Model file for the job. Use its own axes, mm. A direction names the side the tool comes from. Round coordinates to 2 decimals unless told otherwise and drop trailing zeros. Loops run counter-clockwise (first coordinate to the right, second up) from the corner with the lowest first, then second, coordinate; pieces in that order, holes last. Notation, with made-up numbers: M 45.5,72.5 L 86.5,72.5 A18 cw 86.5,104.5 Z; hole C 15.25,51.5 d2. An arc over 180 degrees is marked long. Use a Markdown table: item, result. Add a question column.
Q1. Cut at C-C (z = -9.5). Give the cut face in (x, y), plus the area to 3 significant figures.
Q2. Cut at A-A (x = 12.5). Give the cut face in (y, z).
Q3. Pin check, flat tips, straight feed: pin 1 (5 mm diameter, centred on x = 0, z = 20.5, fed in from +Y); pin 2 (3 mm diameter, centred on x = 20.5, z = 0, fed in from -Y); pin 3 (1 mm diameter, centred on x = 16.5, y = 1.5, fed in from +Z); pin 4 (5 mm diameter, centred on x = 0, z = -9.5, fed in from -Y). Stop position of each tip, or through.
Q4. Probe line 1 (Z direction, x = 0, y = 1.4); line 2 (Z direction, x = 0, y = 1.6); line 3 (X direction, y = 1, z = -13). List the from-to ranges inside material, lowest first. Write a range as from..to.
Q5. Cut at D-D (z = 14). Give the cut face in (x, y).
Q6. Cut at B-B (y = 0.4). State how many separate pieces and enclosed holes the cut face has, plus the area to 3 significant figures.
Q7. Tool access for faces 1 (the face through (4, 2, 4)), 2 (the face through (-16, 1, -3)), 3 (the face through (-3, 1, 16)), 4 (the face through (22.6, 1.01, 2.14)), 5 (the face through (16, 1, -3)): list every direction of +Z, -Z, +X, -X, +Y, -Y with a clear straight run to the whole face (end or side of a thin tool).
Autodesk Inventor part; units mm, degrees
ref_plane "YZ Plane" through (0, 0, 0) normal (1, 0, 0) x (0, 1, 0)
ref_plane "XZ Plane" through (0, 0, 0) normal (0, 1, 0) x (-1, 0, 0)
ref_plane "XY Plane" through (0, 0, 0) normal (0, 0, 1) x (1, 0, 0)
sketch "Skizze1" plane through (0, 0, 0) normal (0, 1, 0) x (-1, 0, 0)
  line L0 (-23.5, -3) -> (23.5, -3)
  line L1 (23.5, -3) -> (23.5, 3)
  line L2 (23.5, 3) -> (-23.5, 3)
  line L3 (-23.5, 3) -> (-23.5, -3)
  line L4 (-23.5, -3) -> (23.5, 3) construction
  line L5 (23.5, -3) -> (-23.5, 3) construction
  line L6 (3, -23.5) -> (-3, -23.5)
  line L7 (-3, -23.5) -> (-3, 23.5)
  line L8 (-3, 23.5) -> (3, 23.5)
  line L9 (3, 23.5) -> (3, -23.5)
  line L10 (3, -23.5) -> (-3, 23.5) construction
  line L11 (-3, -23.5) -> (3, 23.5) construction
  point P0 (0, 0)
  dimension "d0" = 6
  dimension "d1" = 47
extrude "Extrusion1" add sketch "Skizze1" along normal blind 2
sketch "Skizze2" plane through (0, 0, 0) normal (0, -1, 0) x (1, 0, 0)
  circle A0 centre (0, 20.5) radius 1.6
  circle A1 centre (0, -20.5) radius 1.6
  circle A2 centre (20.5, 0) radius 1.6
  circle A3 centre (-20.5, 0) radius 1.6
  line L0 (0, 20.5) -> (0, -20.5) construction
  line L1 (3, -3) -> (3, -23.5) construction
  line L2 (20.5, 0) -> (-20.5, 0) construction
  circle A4 centre (0, 9.5) radius 1.6
  circle A5 centre (0, -9.5) radius 1.6
  circle A6 centre (12.5, 0) radius 1.6
  circle A7 centre (-12.5, 0) radius 1.6
  line L3 (0, 9.5) -> (0, -9.5) construction
  line L4 (12.5, 0) -> (-12.5, 0) construction
  point P0 (0, 0)
  point P1 (0, 0)
  dimension "d4" = 3.2
  dimension "d5" = 41
  dimension "d7" = 19
  dimension "d8" = 25
extrude "Extrusion2" cut sketch "Skizze2" against normal blind 2
fillet "Rundung1" radius 3 8 edges at (-3, 1, 23.5) (3, 1, 23.5) (23.5, 1, 3) (23.5, 1, -3) (3, 1, -23.5) (-3, 1, -23.5) (-23.5, 1, -3) (-23.5, 1, 3)
fillet "Rundung2" radius 8 4 edges at (3, 1, 3) (-3, 1, 3) (-3, 1, -3) (3, 1, -3)
sketch "Skizze3" plane through (0, 0, 0) normal (0, -1, 0) x (1, 0, 0)
  circle A0 centre (0, 0) radius 5
  dimension "d13" = 10
extrude "Extrusion3" cut sketch "Skizze3" against normal blind 2
chamfer "Fase1" distance 1 angle 45 8 edges at (-1.6, 0, 9.5) (-14.1, 0, 0) (10.9, 0, 0) (-1.6, 0, -9.5) (-1.6, 2, 20.5) (-22.1, 2, 0) (18.9, 2, 0) (-1.6, 2, -20.5)
equation "\"G_L\" = 0"
equation "\"G_H\" = 0"
equation "\"G_B\" = 0"
properties part number "Motorkreuz" material "GEDA Stahl"
Checked values:
| question | item | result |
|---|---|---|
| 1 | outline | M -3.14,0 L -2.6,0 L -1.6,1 L -1.6,2 L -3.14,2 Z; M 1.6,1 L 2.6,0 L 3.14,0 L 3.14,2 L 1.6,2 Z |
| 1 | area | 5.17 mm^2 |
| 2 | outline | M 0,-3 L 2,-3 L 2,-1.6 L 1,-1.6 L 0,-2.6 Z; M 0,2.6 L 1,1.6 L 2,1.6 L 2,3 L 0,3 Z |
| 3 | pin 1 | stops at y = 1.9 |
| 3 | pin 2 | passes through |
| 3 | pin 3 | stops at z = 3 |
| 3 | pin 4 | stops at y = 0.1 |
| 4 | line 1 | z = -23.5..-22.5, -18.5..-11.1, -7.9..-5, 5..7.9, 11.1..18.5, 22.5..23.5 |
| 4 | line 2 | z = -23.5..-22.7, -18.3..-11.1, -7.9..-5, 5..7.9, 11.1..18.3, 22.7..23.5 |
| 4 | line 3 | x = -3..3 |
| 5 | outline | M -3,0 L 3,0 L 3,2 L -3,2 Z |
| 6 | separate pieces | 1 |
| 6 | enclosed holes | 9 |
| 6 | area | 396 mm^2 |
| 7 | face 1 | +Z, -Z, +X, -X, +Y |
| 7 | face 2 | -Z, -X, +Y, -Y |
| 7 | face 3 | +Z, -X, +Y, -Y |
| 7 | face 4 | +Z, +X, +Y, -Y |
| 7 | face 5 | -Z, +X, +Y, -Y |
